```python
from build123d import *

# Parameters (mm, degrees)
SKETCH1_R           = 2.75
SKETCH1_W           = 3
SKETCH1_H           = 2.5
BOSS_EXTRUDE1_DEPTH = 2


with BuildPart() as part:
    # Sketch1 → Boss-Extrude1 (new body)
    with BuildSketch(Plane(origin=(0, 0, 0), x_dir=(0, 0, -1), z_dir=(1, 0, 0))):
        with BuildLine():
            Line((30, 10), (0, 10))
            Line((0, 10), (0, 15))
            Line((0, 15), (-30, 15))
            Line((-30, 15), (-30, -15))
            Line((-30, -15), (0, -15))
            Line((0, -15), (0, -10))
            Line((0, -10), (30, -10))
            Line((30, -10), (50.02830583, -5.958427618))
            ThreePointArc((50.02830583, -5.958427618), (56.02830583, 0.041572382), (50.02830583, 6.041572382))
            Line((50.02830583, 6.041572382), (30, 10))
        make_face()
        with Locations((50.02830583, 0.041572382)):
            Circle(SKETCH1_R, mode=Mode.SUBTRACT)
        with Locations((28.5, -6.75)):
            Rectangle(SKETCH1_W, SKETCH1_H, mode=Mode.SUBTRACT)
        with Locations((28.5, -2.25)):
            Rectangle(SKETCH1_W, SKETCH1_H, mode=Mode.SUBTRACT)
        with Locations((28.5, 2.25)):
            Rectangle(SKETCH1_W, SKETCH1_H, mode=Mode.SUBTRACT)
        with Locations((28.5, 6.75)):
            Rectangle(SKETCH1_W, SKETCH1_H, mode=Mode.SUBTRACT)
    extrude(amount=BOSS_EXTRUDE1_DEPTH)


solid = part.part
```
Part model, mm, in its own coordinate system. A direction names the side the tool comes from. Round coordinates to 2 decimals unless told otherwise and drop trailing zeros. Loops run counter-clockwise (first coordinate to the right, second up) from the corner with the lowest first, then second, coordinate; pieces in that order, holes last.
Item 1: Drop flat-ended pins along their axis: P1, Ø0.6, axis at x = 1.5, z = -29, coming from the -Y side; P2, Ø1, axis at x = 1.5, y = 11.5, coming from the -Z side; P3, Ø0.6, axis at x = 0.5, z = -28.5, coming from the +Y side; P4, Ø6, axis at y = -3, z = -39, coming from the -X side. Give the stop position or say it passes through.
Item 2: Mould opens along Y. For faces 1 (the face through (1, -15, 15)), 2 (the face through (1, -7, -27)), 3 (the face through (2, 0, -3)), 4 (the face through (1, 15, 15)) say: +Y half, -Y half, draft (parallel to the pull), parting line (faces both ways), or undercut.
Item 3: Cut at A-A, the plane z = -49. Give the cut face in (x, y), then the cut area to 3 significant figures.
Item 4: Drill centre lines: line 1 (Z direction, x = 1.3, y = -2); line 2 (Z direction, x = 1.7, y = -12.5); line 3 (Y direction, x = 1.4, z = -6). Where is each one in solid material? Low to high.
Item 5: 3-axis set-ups, long thin cutter, end or side, ignore diameter. For faces 5 (the face through (1, 2, -30)), 6 (the face through (1, -13, 0)), 7 (the face through (1, 12, 0)): which of +Z, -Z, +X, -X, +Y, -Y reach the whole face in a straight line?
Item 6: Cut at C-C, the plane z = -9. Give the cut face in (x, y).
Item 7: Cut at B-B, the plane x = 1.05. Give the cut face in (y, z).
A:
1. P1: stops at y = -10
1. P2: stops at z = 0
1. P3: stops at y = 10
1. P4: stops at x = 0
2. face 1: -Y half
2. face 2: undercut
2. face 3: draft
2. face 4: +Y half
3. outline: (0, -6.17) - (2, -6.17) - (2, -2.51) - (0, -2.51) - close; (0, 2.59) - (2, 2.59) - (2, 6.24) - (0, 6.24) - close
3. area: 14.6 mm2
4. line 1: z = -55.67 to -51.87, -48.19 to -30, -27 to 30
4. line 2: z = 0 to 30
4. line 3: y = -10 to 10
5. face 5: +X, -X
5. face 6: -Z, +X, -X, -Y
5. face 7: -Z, +X, -X, +Y
6. outline: (0, -10) - (2, -10) - (2, 10) - (0, 10) - close
7. outline: (-15, 0) - (-10, 0) - (-10, -30) - (-5.96, -50.03) arc R6 ccw to (6.04, -50.03) - (10, -30) - (10, 0) - (15, 0) - (15, 30) - (-15, 30) - close; hole (-8, -30) - (-5.5, -30) - (-5.5, -27) - (-8, -27) - close; hole (-3.5, -30) - (-1, -30) - (-1, -27) - (-3.5, -27) - close; hole circle Ø5.5 at (0.04, -50.03); hole (1, -30) - (3.5, -30) - (3.5, -27) - (1, -27) - close; hole (5.5, -30) - (8, -30) - (8, -27) - (5.5, -27) - close
